Source: CAD feature listing. Evaluate the final solid. Frame: model axes, mm. Face numbers are marked on the shaded views. A direction names the side the tool comes from. Coordinates: 2 decimals unless noted, no trailing zeros. Order: outer loops, then holes, each group sorted by start corner. A loop starts at its lowest first (then second) coordinate and runs counter-clockwise, first axis right, second up. Notation, with made-up numbers: (87.25, 44) -> (106.25, 44) arc R16 cw to (106.25, 59) -> close; hole circle Ø9 at (-29.5, -26). An arc over 180 degrees is marked (long way). Put each result on its own line as item: value.
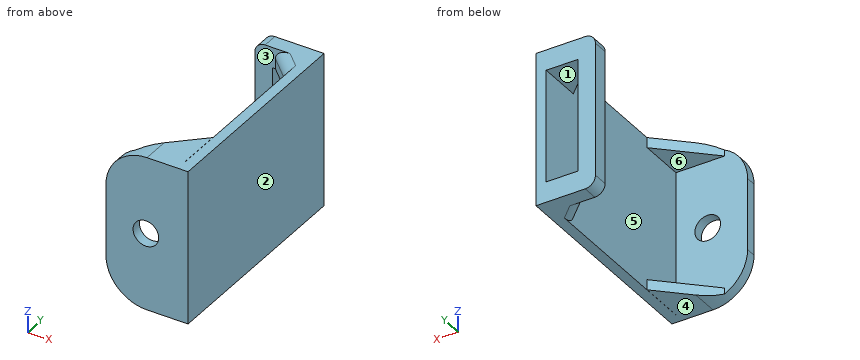
from build123d import *

# Parameters (mm, degrees)
F1_E1_W   = 20.1
F1_E1_H   = 15
F2_DEPTH  = 1
F1_E0_W   = 8
F1_E0_H   = 15
F3_DEPTH  = 1
F5_DEPTH  = 1
F7_DEPTH  = 1
F9_DEPTH  = 1.5
F11_R     = 4
F12_R     = 1
F13_SIZE2 = 2.7039285695
F13_SIZE  = 2.8
F14_R     = 1
F16_D     = 2.5
F16_DEPTH = 3
F16_TIP   = 0.7510757738


with BuildPart() as f2:
    # F1_E1 (on explicit) → F2 (new body)
    with BuildSketch(Plane.YZ):
        with Locations((10.05, 7.5)):
            Rectangle(F1_E1_W, F1_E1_H)
    extrude(amount=-F2_DEPTH)

    # F1_E0 (on explicit) → F3 (join)
    with BuildSketch(Plane(origin=(-8, 0, 0), x_dir=(1, 0, 0), z_dir=(0, -1, 0))):
        with Locations((4, 7.5)):
            Rectangle(F1_E0_W, F1_E0_H)
    extrude(amount=F3_DEPTH)

    # F4 (on Top) → F5 (join)
    with BuildSketch(Plane.XY):
        Polygon((-5.7501993142, 0), (-1.0129548609, 0), (-1.0129548609, 4.4631827623), align=None)
    extrude(amount=F5_DEPTH)

    # F6 (on face) → F7 (join)
    with BuildSketch(Plane.XY.offset(15)):
        Polygon((-5.7530710474, 0), (-1.0158265941, 0), (-1.0158265941, 4.4631827623), align=None)
    extrude(amount=-F7_DEPTH)

    # F8 (on face) → F9 (join)
    with BuildSketch(Plane(origin=(0, 20.1, 0), x_dir=(-1, 0, 0), z_dir=(0, 1, 0))):
        Polygon((5.8, 15), (0, 15), (0, 13), (4.1, 13), (4.1, 2), (0, 2), (0, 0), (5.8, 0), align=None)
    extrude(amount=-F9_DEPTH)

    # F10: union 

    # F11
    f11_edges = [f2.edges().sort_by_distance(p)[0] for p in [
        (-8, -0.5, 0),
        (-8, -0.5, 15),
    ]]
    fillet(f11_edges, radius=F11_R)

    # F12
    f12_edges = [f2.edges().sort_by_distance(p)[0] for p in [
        (-5.8, 19.35, 0),
        (-5.8, 19.35, 15),
    ]]
    fillet(f12_edges, radius=F12_R)

    # F13
    f13_edges = [f2.edges().sort_by_distance(p)[0] for p in [
        (-1, 18.6, 1),
        (-1, 18.6, 14),
    ]]
    chamfer(f13_edges, length=F13_SIZE, length2=F13_SIZE2)

    # F14
    f14_edges = [f2.edges().sort_by_distance(p)[0] for p in [
        (-2.4, 17.248036, 0),
        (-2.4, 17.248036, 15),
    ]]
    fillet(f14_edges, radius=F14_R)

    # F16
    with Locations(Plane.XZ.offset(1)):
        with Locations((-4.1083735414, 7.4923457578)):
            Hole(F16_D / 2, depth=F16_DEPTH)
            with Locations((0, 0, -(F16_DEPTH + F16_TIP / 2))):  # 118° drill point
                Cone(0, F16_D / 2, F16_TIP, mode=Mode.SUBTRACT)


solid = f2.part
1. Cut plane B-B on y = 4. Output: boundary loops of the cut face in (x, z), plus the area to 3 significant figures.
Numbers:
outline: (-1.51, 14) -> (-1.02, 14) -> (-1.02, 15) -> (-1.51, 15) -> close; (-1.5, 0) -> (-1.01, 0) -> (-1.01, 1) -> (-1.5, 1) -> close; (-1, 0) -> (0, 0) -> (0, 15) -> (-1, 15) -> close
area: 16.0 mm2
2. Cut plane D-D on z = 2.75. Output: boundary loops of the cut face in (x, y).
Numbers:
outline: (-7.8, -1) -> (0, -1) -> (0, 20.1) -> (-1, 20.1) -> (-1, 0) -> (-7.8, 0) -> close; (-5.8, 18.6) -> (-4.1, 18.6) -> (-4.1, 20.1) -> (-5.8, 20.1) -> close
3. Set-up query: the marked faces 1 and 2. Return all of +Z, -Z, +X, -X, +Y, -Y with unobstructed straight access to the full face (end or side cutting, diameter ignored); none if empty.
Numbers:
face 1: +Y
face 2: +Z, -Z, +X, +Y, -Y
4. Pull-direction query (Z, two-part tool) for the marked faces 3, 4, 5 and 6; classes: pulls with the +Z half, pulls with the -Z half, needs draft (parallel to the pull), parting line crosses it, or undercut.
Numbers:
face 3: needs draft
face 4: pulls with the -Z half
face 5: undercut
face 6: undercut
5. Ray query, line 1 along Y through (x, z) = (-4.5, 4.5); line 2 along Y through (x, z) = (-6.5, 12.5). Return the intervals inside material, ascending.
Numbers:
line 1: y = -1 to 0, 18.6 to 20.1
line 2: y = -1 to 0
6. First-contact query: pin 1 (8 mm diameter, centred on y = 16.5, z = 8.5, fed in from -X); pin 2 (6 mm diameter, centred on y = 14.5, z = 9.5, fed in from -X); pin 3 (2 mm diameter, centred on x = -4, y = 3.5, fed in from +Z). Flat tips, straight axial feed; report the tip coordinate or a pass-through.
Numbers:
pin 1: stops at x = -5.8
pin 2: stops at x = -1
pin 3: passes through
7. Cut plane C-C on z = 8.25. Output: boundary loops of the cut face in (x, y).
Numbers:
outline: (-8, -1) -> (-5.1, -1) -> (-5.1, 0) -> (-8, 0) -> close; (-5.8, 18.6) -> (-4.1, 18.6) -> (-4.1, 20.1) -> (-5.8, 20.1) -> close; (-3.11, -1) -> (0, -1) -> (0, 20.1) -> (-1, 20.1) -> (-1, 0) -> (-3.11, 0) -> close
8. Cut plane A-A on z = 4.25. Output: boundary loops of the cut face in (x, y), plus the area to 4 significant figures.
Numbers:
outline: (-8, -1) -> (0, -1) -> (0, 20.1) -> (-1, 20.1) -> (-1, 0) -> (-8, 0) -> close; (-5.8, 18.6) -> (-4.1, 18.6) -> (-4.1, 20.1) -> (-5.8, 20.1) -> close
area: 30.65 mm2
